Could you check a few things on this model? Use its own coordinates, in mm. A direction names the side the tool comes from. Coordinates: 2 decimals unless noted, no trailing zeros. Write each loop counter-clockwise with the first axis right and the second up, starting at its lowest first coordinate (ties: lowest second). Pieces come first, ordered by that corner, then holes. Notation, with made-up numbers: (-27.5, -31.5) - (13.5, -31.5) arc R28 ccw to (13.5, 4.5) - close; hole circle Ø11 at (29.5, 31). An arc over 180 degrees is marked (long way). Answer as a JSON object with one key per item and string values. Group by question number.
1) If we section it at D-D (x = 20.5): Write out the boundary of the cut face in (y, z) (3 decimals).
2) Will these pins go through, and if not, where does the flat tip stop? pin 1 Ø2.5 at (x, y) = (0, 9.525) entering from +Z; pin 2 Ø2 at (x, y) = (-15, 7.5) entering from -Z (3 decimals); pin 3 Ø2 at (x, y) = (23.35, 23.35) entering from +Z; pin 4 Ø2 at (x, y) = (0, -9.525) entering from +Z (3 decimals).
3) On a 3-axis mill with a long thin cutter (end or side, diameter ignored), from which of +Z, -Z, +X, -X, +Y, -Y can I reach the whole of each face in a straight line? I mean faces 1 (the cylindrical face through (0.499, -10.484, 3.425)), 2 (the flat face through (25.4, 25.4, 3.4)). Say none if no direction works.
4) If we section it at B-B (y = 13.97): Write out the boundary of the cut face in (x, z) (1 decimal).
5) If we section it at C-C (x = 0): State how many separate pieces and enclosed holes the cut face has, plus the area to 3 significant figures.
6) Please list where these lines run through material, in increasing order: line 1 along Y through (x, z) = (0, 3.5); line 2 along X through (y, z) = (-5.5, 3.5); line 3 along Y through (x, z) = (-24, 3.25) (3 decimals).
7) We'd pull the mould along Y, two halves only. Please class faces 3 (the flat face through (3.4, -5.2, 3.175)), 4 (the flat face through (-12, 0, 3.175)), 5 (the cylindrical face through (10.902, 3.433, 1.565)): released by +Y, released by -Y, zero draft, split by the parting line, or undercut.
8) If we section it at A-A (y = 0): Write out the boundary of the cut face in (x, z) (1 decimal), plus the area to 3 significant figures.
```python
from build123d import *

# Parameters (mm, degrees)
SKETCH1_R             = 11.43
SKETCH1_R_2           = 5.08
BOSS_EXTRUDE1_DEPTH   = 3.175
FILLET1_R             = 0.635
F_2_56_TAPPED_HOLE1_D = 1.778
SKETCH4_W             = 53.34
SKETCH4_H             = 53.34
SKETCH4_R             = 7.9375
SKETCH4_R_2           = 1.084817848
SKETCH4_R_3           = 1.08040081
BOSS_EXTRUDE2_DEPTH   = 0.508
F_4_CLEARANCE_HOLE1_D = 3.2639
CIRPATTERN1_COUNT     = 4
SKETCH9_R             = 1.5875
CUT_EXTRUDE1_DEPTH    = 0.508
CHAMFER1_SIZE         = 2.54


with BuildPart() as part:
    # Sketch1 → Boss-Extrude1 (new body)
    with BuildSketch(Plane.XY):
        Circle(SKETCH1_R)
        Circle(SKETCH1_R_2, mode=Mode.SUBTRACT)
    extrude(amount=BOSS_EXTRUDE1_DEPTH)

    # Fillet1
    fillet1_edges = [part.edges().sort_by_distance(p)[0] for p in [
        (-5.08, 0, 0),
        (-5.08, 0, 3.175),
    ]]
    fillet(fillet1_edges, radius=FILLET1_R)

    # #2-56 Tapped Hole1 (through all)
    with Locations(Plane.XY.offset(3.175)):
        with Locations((0, 9.525)):
            f_2_56_tapped_hole1 = Hole(F_2_56_TAPPED_HOLE1_D / 2)

    # Mirror1: #2-56 Tapped Hole1 across plane
    add(f_2_56_tapped_hole1.mirror(Plane.ZX), mode=Mode.SUBTRACT)

    # Sketch4 → Boss-Extrude2 (add)
    with BuildSketch(Plane.XY.offset(3.175)):
        Rectangle(SKETCH4_W, SKETCH4_H)
        Circle(SKETCH4_R, mode=Mode.SUBTRACT)
        with Locations((0, 9.525)):
            Circle(SKETCH4_R_2, mode=Mode.SUBTRACT)
        with Locations((0, -9.525)):
            Circle(SKETCH4_R_3, mode=Mode.SUBTRACT)
    extrude(amount=BOSS_EXTRUDE2_DEPTH)

    # #4 Clearance Hole1 (through all)
    with Locations(Plane(origin=(0, 0, 3.175), x_dir=(-1, 0, 0), z_dir=(0, 0, -1))):
        with Locations((-23.348665915, -23.348665915)):
            f_4_clearance_hole1 = Hole(F_4_CLEARANCE_HOLE1_D / 2)

    # CirPattern1: #4 Clearance Hole1 ×4 about axis
    cirpattern1_axis = Axis((0, 0, 0), (0, 0, 1))
    for i in range(1, CIRPATTERN1_COUNT):
        add(f_4_clearance_hole1.rotate(cirpattern1_axis, i * 360 / CIRPATTERN1_COUNT), mode=Mode.SUBTRACT)

    # Sketch9 → Cut-Extrude1 (cut)
    with BuildSketch(Plane.XY.offset(3.683)):
        with Locations((0, 13.97)):
            Circle(SKETCH9_R)
    extrude(amount=-CUT_EXTRUDE1_DEPTH, mode=Mode.SUBTRACT)

    # Chamfer1
    chamfer1_edges = [part.edges().sort_by_distance(p)[0] for p in [
        (-26.67, 26.67, 3.429),
        (-26.67, -26.67, 3.429),
        (26.67, -26.67, 3.429),
        (26.67, 26.67, 3.429),
    ]]
    chamfer(chamfer1_edges, length=CHAMFER1_SIZE)


solid = part.part
```
Here are the results:
{
 "1": {"outline": "(-26.67, 3.175) - (26.67, 3.175) - (26.67, 3.683) - (-26.67, 3.683) - close"},
 "2": {"pin 1": "stops at z = 3.68", "pin 2": "stops at z = 3.175", "pin 3": "passes through", "pin 4": "stops at z = 3.175"},
 "3": {"face 1": "+Z", "face 2": "+Z, -Z, +X, +Y"},
 "4": {"outline": "(-26.7, 3.2) - (-1.6, 3.2) - (-1.6, 3.7) - (-26.7, 3.7) - close; (1.6, 3.2) - (26.7, 3.2) - (26.7, 3.7) - (1.6, 3.7) - close"},
 "5": {"separate pieces": "5", "enclosed holes": "0", "area": "43.9 mm²"},
 "6": {"line 1": "y = -26.67 to -10.61, -8.44 to -7.94, 7.94 to 8.44, 10.61 to 12.38, 15.56 to 26.67", "line 2": "x = -26.67 to -5.72, 5.72 to 26.67", "line 3": "y = -26.67 to -24.845, -21.852 to 21.852, 24.845 to 26.67"},
 "7": {"face 3": "undercut", "face 4": "zero draft", "face 5": "split by the parting line"},
 "8": {"outline": "(-26.7, 3.2) - (-11.4, 3.2) - (-11.4, 0) - (-5.7, 0) arc R0.6 ccw to (-5.1, 0.6) - (-5.1, 2.5) arc R0.6 ccw to (-5.7, 3.2) - (-7.9, 3.2) - (-7.9, 3.7) - (-26.7, 3.7) - close; (5.1, 0.6) arc R0.6 ccw to (5.7, 0) - (11.4, 0) - (11.4, 3.2) - (26.7, 3.2) - (26.7, 3.7) - (7.9, 3.7) - (7.9, 3.2) - (5.7, 3.2) arc R0.6 ccw to (5.1, 2.5) - close", "area": "59.0 mm²"}
}
